Input: dimensioned drawing with shaded views. Units: mm. Origin: part minimum x, y, z. A direction names the side the tool comes from. Give positions to 0.01 mm unless a question says otherwise; leave off trailing zeros. Write each loop counter-clockwise with the first axis right and the second up, starting at its lowest first coordinate (ties: lowest second). Pieces come first, ordered by that corner, then holes.
Q1. Section B-B (y = 4). Return the cut outline in (x, z).
Q2. Reachability of the marked faces 1 and 2 from +Z, -Z, +X, -X, +Y, -Y: full face, straight path, thin tool, end or side. Return the list, or none.
Q3. Pin query (flat end, axial travel): pin 1 Ø0.5 at (x, y) = (1, 0.5) entering from +Z; pin 2 Ø0.5 at (y, z) = (0.5, 4.5) entering from +X; pin 3 Ø2.5 at (x, z) = (6, 5.5) entering from -Y; pin 4 Ø0.5 at (y, z) = (0.5, 4.5) entering from -X. Return the tip coordinate at first contact, or that it passes through.
Q4. Section A-A (x = 5). Return the cut outline in (y, z).
Q5. Section D-D (x = 1). Return the cut outline in (y, z), plus the area to 3 significant figures.
Q6. Section C-C (z = 5). Return the cut outline in (x, y), plus the area to 3 significant figures.
Q7. Line query: line 1 (Y direction, x = 9.5, z = 4.5); line 2 (Y direction, x = 3.75, z = 5); line 3 (X direction, y = 13.5, z = 1.25) (1 decimal). Output: solid intervals per line, ascending.
Q8. Mould query, pull axis X, two halves, no side actions, for the marked faces 3, 4 and 5. Classes: +X half, -X half, draft (parallel to the pull), parting line (faces both ways), or undercut.
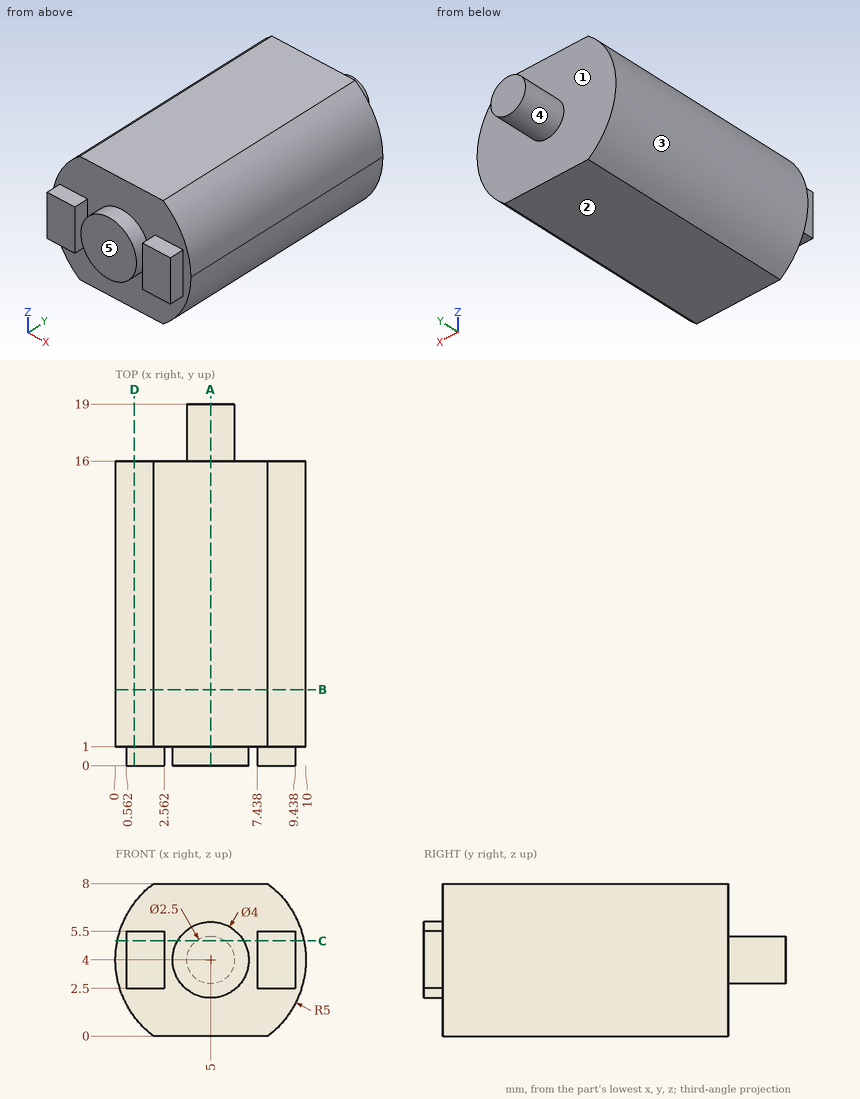
Computed:
1. outline: (2, 0) - (8, 0) arc R5 ccw to (8, 8) - (2, 8) arc R5 ccw to start
2. face 1: +Y
2. face 2: -Z, +X, -X, +Y, -Y
3. pin 1: stops at z = 5.5
3. pin 2: stops at x = 9.44
3. pin 3: stops at y = 0
3. pin 4: stops at x = 0.56
4. outline: (0, 2) - (1, 2) - (1, 0) - (16, 0) - (16, 2.75) - (19, 2.75) - (19, 5.25) - (16, 5.25) - (16, 8) - (1, 8) - (1, 6) - (0, 6) - close
5. outline: (0, 2.5) - (1, 2.5) - (1, 1) - (16, 1) - (16, 7) - (1, 7) - (1, 5.5) - (0, 5.5) - close
5. area: 93.0 mm2
6. outline: (0.1, 1) - (0.56, 1) - (0.56, 0) - (2.56, 0) - (2.56, 1) - (3.27, 1) - (3.27, 0) - (6.73, 0) - (6.73, 1) - (7.44, 1) - (7.44, 0) - (9.44, 0) - (9.44, 1) - (9.9, 1) - (9.9, 16) - (5.75, 16) - (5.75, 19) - (4.25, 19) - (4.25, 16) - (0.1, 16) - close
6. area: 159 mm2
7. line 1: y = 1 to 16
7. line 2: y = 0 to 16
7. line 3: x = 0.8 to 9.2
8. face 3: -X half
8. face 4: parting line
8. face 5: draft
